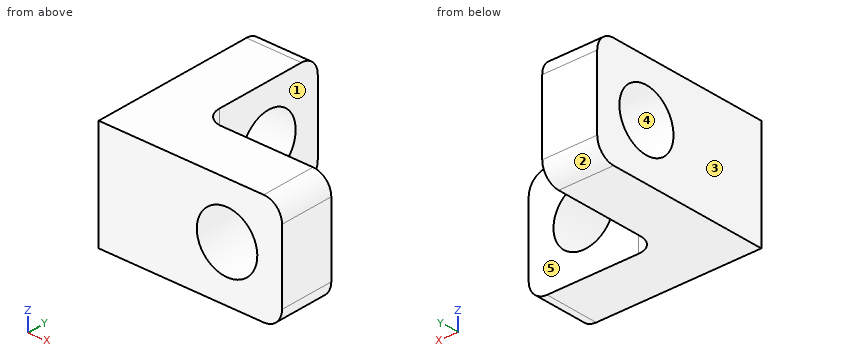
from build123d import *

# Parameters (mm, degrees)
EXTRUDE_1_DEPTH     = 6
SKETCH_2_R          = 1.65
CUT_EXTRUDE_1_DEPTH = 6
SKETCH_3_R          = 1.65
CUT_EXTRUDE_2_DEPTH = 6
FILLET_1_R          = 1


with BuildPart() as part:
    # 草图1 → 凸台-拉伸1 (new body)
    with BuildSketch(Plane.XY):
        Polygon((10, 0), (0, 0), (0, 10), (3, 10), (3, 3), (10, 3), align=None)
    extrude(amount=EXTRUDE_1_DEPTH)

    # 草图2 → 切除-拉伸1 (cut)
    with BuildSketch(Plane(origin=(3, 0, 0), x_dir=(0, 0, -1), z_dir=(1, 0, 0))):
        with Locations(Location((-3, 7, 0), (0, 0, 90))):
            Circle(SKETCH_2_R)
    extrude(amount=-CUT_EXTRUDE_1_DEPTH, mode=Mode.SUBTRACT)

    # 草图3 → 切除-拉伸2 (cut)
    with BuildSketch(Plane(origin=(0, 3, 0), x_dir=(1, 0, 0), z_dir=(0, 1, 0))):
        with Locations(Location((7, -3, 0), (0, 0, 270))):
            Circle(SKETCH_3_R)
    extrude(amount=-CUT_EXTRUDE_2_DEPTH, mode=Mode.SUBTRACT)

    # 圆角1
    fillet_1_edges = [part.edges().sort_by_distance(p)[0] for p in [
        (3, 3, 3),
        (1.5, 10, 6),
        (10, 1.5, 6),
        (1.5, 10, 0),
        (10, 1.5, 0),
    ]]
    fillet(fillet_1_edges, radius=FILLET_1_R)


solid = part.part
The listing builds one solid part. Answer for the finished solid, in the listing's coordinates (mm). Face numbers are marked on the shaded views. A direction names the side the tool comes from. Give positions to 0.01 mm unless a question says otherwise; leave off trailing zeros. Write each loop counter-clockwise with the first axis right and the second up, starting at its lowest first coordinate (ties: lowest second). Pieces come first, ordered by that corner, then holes.
1) For a pull along Y with two mould halves and no side action, classify the marked faces 3, 4 and 5 as pulls with the +Y half, pulls with the -Y half, needs draft (parallel to the pull), parting line crosses it, or undercut.
2) Find the intervals of material crossed by L1, parallel to X at y = 1.6, z = 3; L2, parallel to Z at x = 1.6, y = 7; L3, parallel to X at y = 7, z = 5.55, in increasing order.
3) Section D-D (z = 1.7) is taken. Write down the section's boundary in (x, y).
4) Section B-B (y = 7) is taken. Write down the section's boundary in (x, z), and give its area (3 significant figures).
5) Given P1, Ø3, axis at y = 7, z = 2, coming from the +X side; P2, Ø1.8, axis at x = 5.5, z = 2.5, coming from the +Y side; P3, Ø2, axis at y = 8, z = 2.5, coming from the -X side, each flat-ended and moving along its own axis, determine where each tip first touches the part or whether it passes through.
6) Section A-A (z = 3) is taken. Write down the section's boundary in (x, y), and give its area (3 significant figures).
7) A tool of negligible diameter and unlimited length cuts with its end or side. For the marked faces 1 and 2, from which of +Z, -Z, +X, -X, +Y, -Y can it reach the whole face along a straight path? Write none if from no direction.
Response:
1. face 3: needs draft
1. face 4: undercut
1. face 5: pulls with the +Y half
2. L1: x = 0 to 5.35, 8.65 to 10
2. L2: z = 0 to 1.35, 4.65 to 6
2. L3: x = 0 to 3
3. outline: (0, 0) - (5.98, 0) - (5.98, 3) - (4, 3) arc R1 cw to (3, 4) - (3, 5.98) - (0, 5.98) - close; (0, 8.02) - (3, 8.02) - (3, 10) - (0, 10) - close; (8.02, 0) - (10, 0) - (10, 3) - (8.02, 3) - close
4. outline: (0, 0) - (3, 0) - (3, 1.35) - (0, 1.35) - close; (0, 4.65) - (3, 4.65) - (3, 6) - (0, 6) - close
4. area: 8.10 mm2
5. P1: stops at x = 3
5. P2: stops at y = 3
5. P3: stops at x = 0
6. outline: (0, 0) - (5.35, 0) - (5.35, 3) - (4, 3) arc R1 cw to (3, 4) - (3, 5.35) - (0, 5.35) - close; (0, 8.65) - (3, 8.65) - (3, 10) - (0, 10) - close; (8.65, 0) - (10, 0) - (10, 3) - (8.65, 3) - close
6. area: 31.4 mm2
7. face 1: +Z, -Z, +X, +Y
7. face 2: -Z, +X, -X, +Y
